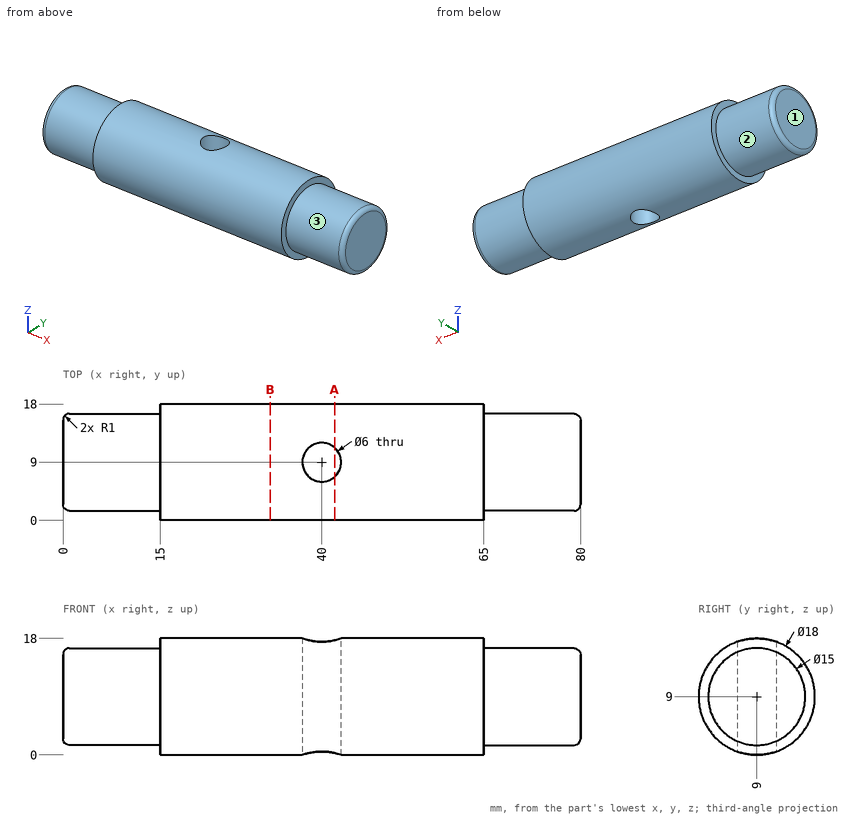
Print and shaded views of the part. All mm, measured from the part's lowest x, y and z. A direction names the side the tool comes from. Give positions to 0.01 mm unless a question says otherwise; leave off trailing zeros. Loops run counter-clockwise (first coordinate to the right, second up) from the corner with the lowest first, then second, coordinate; pieces in that order, holes last. Notation, with made-up numbers: M -35,49 L 3,49 A29 cw 3,72 Z; hole C 29.5,-37 d6. An arc over 180 degrees is marked long. Write each question's results on one line, items separated by ' | '.
Q1. Band-saw the part on A-A on x = 42. Write the cut outline in (y, z).
Geometry check:
outline: M 6.76,0.28 L 6.76,17.72 A9 ccw Z; M 11.24,0.28 A9 ccw 11.24,17.72 Z
Q2. Band-saw the part on B-B on x = 32. Write the cut outline in (y, z), and give its area (3 significant figures).
Geometry check:
outline: C 9,9 d18 | area: 254 mm²
Q3. Flat gauge pins, fed straight in: P1, Ø3.5, axis at x = 40, y = 9, coming from the +Z side; P2, Ø1, axis at x = 51.5, z = 12.5, coming from the +Y side; P3, Ø8, axis at x = 24.5, y = 2.5, coming from the -Z side; P4, Ø5, axis at x = 37.5, y = 13.5, coming from the -Z side. Where does each tip first touch, or does it go through?
Geometry check:
P1: passes through | P2: stops at y = 17.49 | P3: stops at z = 0.35 | P4: stops at z = 0.23
Q4. Probe probe 1 along Y at (x, z) = (40, 5); probe 2 along X at (y, z) = (9.5, 14.25); probe 3 along X at (y, z) = (14.25, 15). List the from-to ranges inside material, lowest first.
Geometry check:
probe 1: y = 0.94 to 6, 12 to 17.06 | probe 2: x = 0 to 37.04, 42.96 to 80 | probe 3: x = 15 to 65
Q5. Which spindle directions (+Z, -Z, +X, -X, +Y, -Y) get a long thin tool onto all of the face, cutting with end or side? Do the marked faces 1, 2 and 3. Say none if no direction does.
Geometry check:
face 1: +Z, -Z, -X, +Y, -Y | face 2: -X | face 3: +X
